```python
from build123d import *

# Parameters (mm, degrees)
SKETCH1_W           = 66.04
SKETCH1_H           = 38.1
BOSS_EXTRUDE3_DEPTH = 17.78
SKETCH3_W           = 60.96
SKETCH3_H           = 33.02
CUT_EXTRUDE1_DEPTH  = 15.24
SKETCH4_W           = 38.1
SKETCH4_H           = 8.89
CUT_EXTRUDE2_DEPTH  = 66.04
SKETCH5_R           = 0.635
CUT_EXTRUDE3_DEPTH  = 5.08


with BuildPart() as part:
    # Sketch1 → Boss-Extrude3 (new body)
    with BuildSketch(Plane(origin=(0, 0, 0), x_dir=(1, 0, 0), z_dir=(0, 1, 0))):
        with Locations((33.02, 19.05)):
            Rectangle(SKETCH1_W, SKETCH1_H)
    extrude(amount=BOSS_EXTRUDE3_DEPTH)

    # Sketch3 → Cut-Extrude1 (cut)
    with BuildSketch(Plane(origin=(0, 17.78, 0), x_dir=(1, 0, 0), z_dir=(0, 1, 0))):
        with Locations((33.02, 19.05)):
            Rectangle(SKETCH3_W, SKETCH3_H)
    extrude(amount=-CUT_EXTRUDE1_DEPTH, mode=Mode.SUBTRACT)

    # Sketch4 → Cut-Extrude2 (cut)
    with BuildSketch(Plane(origin=(66.04, 0, 0), x_dir=(0, 0, -1), z_dir=(1, 0, 0))):
        with Locations((19.05, 13.335)):
            Rectangle(SKETCH4_W, SKETCH4_H)
    extrude(amount=-CUT_EXTRUDE2_DEPTH, mode=Mode.SUBTRACT)

    # Sketch5 → Cut-Extrude3 (cut)
    with BuildSketch(Plane(origin=(0, 8.89, 0), x_dir=(1, 0, 0), z_dir=(0, 1, 0))):
        with Locations((33.02, 36.83)):
            Circle(SKETCH5_R)
        with Locations((33.02, 1.27)):
            Circle(SKETCH5_R)
        with Locations((1.27, 19.05)):
            Circle(SKETCH5_R)
        with Locations((64.77, 19.05)):
            Circle(SKETCH5_R)
    extrude(amount=-CUT_EXTRUDE3_DEPTH, mode=Mode.SUBTRACT)


solid = part.part
```
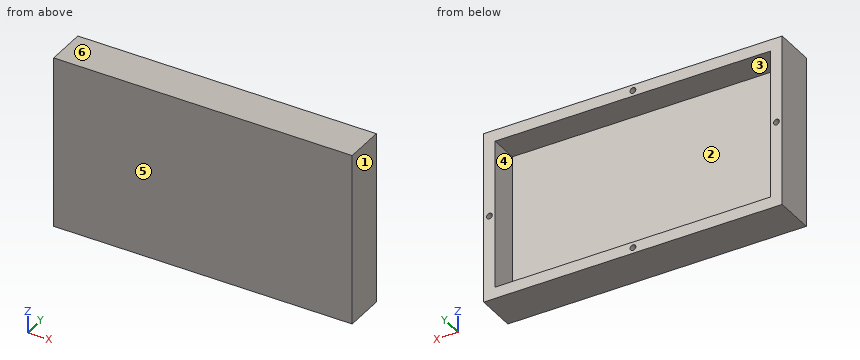
The listing builds one solid part. Answer for the finished solid, in the listing's coordinates (mm). Face numbers are marked on the shaded views. A direction names the side the tool comes from. Give positions to 0.01 mm unless a question says otherwise; leave off trailing zeros. Order: outer loops, then holes, each group sorted by start corner. A loop starts at its lowest first (then second) coordinate and runs counter-clockwise, first axis right, second up. Notation, with made-up numbers: (-20, 1.25) -> (12, 1.25) arc R21 cw to (12, 12.25) -> close; hole circle Ø1 at (82, 25.25). An arc over 180 degrees is marked (long way). One line per item, written item: value.
1) Find section C-C, the plane z = -25. Determine the outline of the cut face in (x, y), plus the area to 3 significant figures.
Reported:
outline: (0, 0) -> (66.04, 0) -> (66.04, 8.89) -> (63.5, 8.89) -> (63.5, 2.54) -> (2.54, 2.54) -> (2.54, 8.89) -> (0, 8.89) -> close
area: 200 mm^2
2) Find section B-B, the plane x = 64.77. Determine the outline of the cut face in (y, z) (3 decimals), plus the area to 3 significant figures.
Reported:
outline: (0, -38.1) -> (8.89, -38.1) -> (8.89, -19.685) -> (3.81, -19.685) -> (3.81, -18.415) -> (8.89, -18.415) -> (8.89, 0) -> (0, 0) -> close
area: 332 mm^2
3) Find the intervals of material crossed by line 1 (X direction, y = 6.15, z = -19.05) (3 decimals); line 2 (X direction, y = 6.85, z = -36.83) (3 decimals); line 3 (X direction, y = 5.25, z = -3.5), in increasing order.
Reported:
line 1: x = 0 to 0.635, 1.905 to 2.54, 63.5 to 64.135, 65.405 to 66.04
line 2: x = 0 to 32.385, 33.655 to 66.04
line 3: x = 0 to 2.54, 63.5 to 66.04
4) A tool of negligible diameter and unlimited length cuts with its end or side. For the marked faces 1 and 2, from which of +Z, -Z, +X, -X, +Y, -Y can it reach the whole face along a straight path? Write none if from no direction.
Reported:
face 1: +Z, -Z, +X, +Y, -Y
face 2: +Y
5) Determine the mould class of the marked faces 3, 4, 5 and 6 for opening direction Z: pulls with the +Z half, pulls with the -Z half, needs draft (parallel to the pull), parting line crosses it, or undercut.
Reported:
face 3: undercut
face 4: undercut
face 5: needs draft
face 6: pulls with the +Z half
6) Find section D-D, the plane z = -19.05. Determine the outline of the cut face in (x, y) (3 decimals).
Reported:
outline: (0, 0) -> (66.04, 0) -> (66.04, 8.89) -> (65.405, 8.89) -> (65.405, 3.81) -> (64.135, 3.81) -> (64.135, 8.89) -> (63.5, 8.89) -> (63.5, 2.54) -> (2.54, 2.54) -> (2.54, 8.89) -> (1.905, 8.89) -> (1.905, 3.81) -> (0.635, 3.81) -> (0.635, 8.89) -> (0, 8.89) -> close
7) Find section A-A, the plane y = 5.5. Determine the outline of the cut face in (x, z) (3 decimals).
Reported:
outline: (0, -38.1) -> (66.04, -38.1) -> (66.04, 0) -> (0, 0) -> close; hole circle Ø1.27 at (1.27, -19.05); hole (2.54, -35.56) -> (63.5, -35.56) -> (63.5, -2.54) -> (2.54, -2.54) -> close; hole circle Ø1.27 at (33.02, -36.83); hole circle Ø1.27 at (33.02, -1.27); hole circle Ø1.27 at (64.77, -19.05)
8) Flat-ended cylindrical pins translate along their axes: P1, Ø2, axis at x = 51, z = -34, coming from the +Y side; P2, Ø0.8, axis at x = 33.02, z = -36.83, coming from the +Y side. Find the tip coordinate at first contact, or state that the pin passes through.
Reported:
P1: stops at y = 2.54
P2: stops at y = 3.81
